Design review of the part built by this model. Coordinates are the model's own, in mm. A direction names the side the tool comes from. Give positions to 0.01 mm unless a question says otherwise; leave off trailing zeros. Loops run counter-clockwise (first coordinate to the right, second up) from the corner with the lowest first, then second, coordinate; pieces in that order, holes last. Notation, with made-up numbers: (39.5, 0.25) - (48.5, 0.25) arc R20 ccw to (48.5, 24.25) - close; hole circle Ø9 at (15.5, 74.5). An arc over 180 degrees is marked (long way). Write each question's results on one line, items separated by ' | '.
from build123d import *

# Parameters (mm, degrees)
SKETCH1_W           = 15.62
SKETCH1_H           = 19.43
BOSS_EXTRUDE1_DEPTH = 2.29
SKETCH2_W           = 11.43
SKETCH2_H           = 11.43
BOSS_EXTRUDE2_DEPTH = 3.81
FILLET1_R           = 1
SKETCH3_W           = 12.5
SKETCH3_H           = 15
BOSS_EXTRUDE3_DEPTH = 9.4
SKETCH4_W           = 5.08
SKETCH4_H           = 8.13
BOSS_EXTRUDE4_DEPTH = 8.13


with BuildPart() as part:
    # Sketch1 → Boss-Extrude1 (new body)
    with BuildSketch(Plane.XY):
        Rectangle(SKETCH1_W, SKETCH1_H)
    extrude(amount=BOSS_EXTRUDE1_DEPTH)

    # Sketch2 → Boss-Extrude2 (add)
    with BuildSketch(Plane(origin=(0, 0, 0), x_dir=(-1, 0, 0), z_dir=(0, 0, -1))):
        Rectangle(SKETCH2_W, SKETCH2_H)
    extrude(amount=-BOSS_EXTRUDE2_DEPTH)

    # Fillet1
    fillet1_edges = [part.edges().sort_by_distance(p)[0] for p in [
        (-7.81, 0, 2.29),
        (0, -9.715, 2.29),
        (7.81, 0, 2.29),
        (0, 9.715, 2.29),
    ]]
    fillet(fillet1_edges, radius=FILLET1_R)

    # Sketch3 → Boss-Extrude3 (add)
    with BuildSketch(Plane(origin=(0, 0, 0), x_dir=(-1, 0, 0), z_dir=(0, 0, -1))):
        Rectangle(SKETCH3_W, SKETCH3_H)
    extrude(amount=BOSS_EXTRUDE3_DEPTH)

    # Sketch4 → Boss-Extrude4 (add)
    with BuildSketch(Plane(origin=(0, 0, -9.4), x_dir=(-1, 0, 0), z_dir=(0, 0, -1))):
        Rectangle(SKETCH4_W, SKETCH4_H)
    extrude(amount=BOSS_EXTRUDE4_DEPTH)


solid = part.part
(1) Insertion check: P1, Ø4.5, axis at y = -3, z = -5.5, coming from the -X side; P2, Ø4, axis at x = -1, z = -11.5, coming from the -Y side (3 decimals); P3, Ø0.5, axis at x = -1, z = 3, coming from the +Y side (3 decimals); P4, Ø1, axis at y = -5.5, z = -15.5, coming from the +X side. Each pin has a flat end and moves straight along its axis. Give the tip position at first contact, or say it passes through.
Answers below:
P1: x = -6.25 | P2: y = -4.065 | P3: y = 5.715 | P4: through
(2) Take a section at A-A on x = 3.25. Give the boundary of the cut face in (y, z) (3 decimals).
Answers below:
outline: (-9.715, 0) - (-7.5, 0) - (-7.5, -9.4) - (7.5, -9.4) - (7.5, 0) - (9.715, 0) - (9.715, 1.29) arc R1 ccw to (8.715, 2.29) - (5.715, 2.29) - (5.715, 3.81) - (-5.715, 3.81) - (-5.715, 2.29) - (-8.715, 2.29) arc R1 ccw to (-9.715, 1.29) - close
(3) Take a section at B-B on y = 7. Give the boundary of the cut face in (x, z), plus the area to 3 significant figures.
Answers below:
outline: (-7.81, 0) - (-6.25, 0) - (-6.25, -9.4) - (6.25, -9.4) - (6.25, 0) - (7.81, 0) - (7.81, 1.29) arc R1 ccw to (6.81, 2.29) - (-6.81, 2.29) arc R1 ccw to (-7.81, 1.29) - close | area: 153 mm2
(4) Take a section at D-D on y = 1.25. Give the boundary of the cut face in (x, z) (3 decimals).
Answers below:
outline: (-7.81, 0) - (-6.25, 0) - (-6.25, -9.4) - (-2.54, -9.4) - (-2.54, -17.53) - (2.54, -17.53) - (2.54, -9.4) - (6.25, -9.4) - (6.25, 0) - (7.81, 0) - (7.81, 1.29) arc R1 ccw to (6.81, 2.29) - (5.715, 2.29) - (5.715, 3.81) - (-5.715, 3.81) - (-5.715, 2.29) - (-6.81, 2.29) arc R1 ccw to (-7.81, 1.29) - close
(5) Tool access review of faces 1 (the flat face through (2.54, 0, -13)), 2 (the flat face through (-5.715, 0, 3)), 3 (the flat face through (5.715, 0, 3)), 4 (the flat face through (-6.25, 0, -5)), 5 (the flat face through (0, -7.5, -5)): name each direction out of +Z, -Z, +X, -X, +Y, -Y from which nothing blocks a thin tool from reaching the whole face with its end or side.
Answers below:
face 1: -Z, +X, +Y, -Y | face 2: +Z, -X, +Y, -Y | face 3: +Z, +X, +Y, -Y | face 4: -Z, -X, +Y, -Y | face 5: -Z, +X, -X, -Y
(6) Wall thickness on line 1 along Y through (x, z) = (6, -7.25); line 2 along Y through (x, z) = (-2.5, -12.5) (3 decimals); line 3 along Z through (x, y) = (6, -8): over which ranges is each line inside the solid? List them lowest first. Write a range as from..to.
Answers below:
line 1: -7.5..7.5 | line 2: -4.065..4.065 | line 3: 0..2.29
(7) Take a section at C-C on z = -9.75. Give the boundary of the cut face in (x, y) (3 decimals).
Answers below:
outline: (-2.54, -4.065) - (2.54, -4.065) - (2.54, 4.065) - (-2.54, 4.065) - close
